Autodesk Inventor part; units mm, degrees
ref_plane "YZ Plane" through (0, 0, 0) normal (1, 0, 0) x (0, 1, 0)
ref_plane "XZ Plane" through (0, 0, 0) normal (0, 1, 0) x (-1, 0, 0)
ref_plane "XY Plane" through (0, 0, 0) normal (0, 0, 1) x (1, 0, 0)
sketch "Sketch1" plane through (0, 0, 0) normal (0, 1, 0) x (-1, 0, 0)
  line L0 (-30, -43) -> (30, -43)
  line L1 (30, -43) -> (30, 43)
  line L2 (30, 43) -> (-30, 43)
  line L3 (-30, 43) -> (-30, -43)
  line L4 (-30, -43) -> (30, 43) construction
  line L5 (30, -43) -> (-30, 43) construction
  line L6 (0, 43) -> (0, 45)
  line L7 (30, 0) -> (32, 0)
  line L8 (-30, -45) -> (30, -45)
  line L9 (32, -43) -> (32, 43)
  line L10 (30, 45) -> (-30, 45)
  line L11 (-32, 43) -> (-32, -43)
  line L12 (-32, -45) -> (32, 45) construction
  line L13 (32, -45) -> (-32, 45) construction
  arc A0 (-32, -43) -> (-30, -45) centre (-30, -43) ccw
  arc A1 (30, -45) -> (32, -43) centre (30, -43) ccw
  arc A2 (32, 43) -> (30, 45) centre (30, 43) ccw
  arc A3 (-30, 45) -> (-32, 43) centre (-30, 43) ccw
  point P0 (0, 0)
  dimension "d0" = 60
  dimension "d1" = 86
  dimension "d3" = 2
  dimension "d4" = 2
  dimension "d26" = 2
extrude "Extrusion1" add sketch "Sketch1" along normal blind 2
sketch "Sketch2" plane through (0, 2, 0) normal (0, 1, 0) x (1, 0, 0)
  line L0 (-30, -43) -> (30, -43)
  line L1 (30, -43) -> (30, 43)
  line L2 (30, 43) -> (-30, 43)
  line L3 (-30, 43) -> (-30, -43)
  line L4 (-30, -43) -> (30, 43) construction
  line L5 (30, -43) -> (-30, 43) construction
  line L6 (0, 43) -> (0, 45)
  line L7 (30, 0) -> (32, 0)
  line L8 (-30, -45) -> (30, -45)
  line L9 (32, -43) -> (32, 43)
  line L10 (30, 45) -> (-30, 45)
  line L11 (-32, 43) -> (-32, -43)
  line L12 (-32, -45) -> (32, 45) construction
  line L13 (32, -45) -> (-32, 45) construction
  arc A0 (32, 43) -> (30, 45) centre (30, 43) ccw
  arc A1 (-30, 45) -> (-32, 43) centre (-30, 43) ccw
  arc A2 (-32, -43) -> (-30, -45) centre (-30, -43) ccw
  arc A3 (30, -45) -> (32, -43) centre (30, -43) ccw
  point P0 (0, 0)
  point P1 (0, 0)
  dimension "d7" = 60
  dimension "d8" = 86
  dimension "d9" = 2
  dimension "d10" = 2
  dimension "d27" = 2
extrude "Extrusion2" add sketch "Sketch2" along normal blind 55 contours L0 L1 L7 L9 A3 L8 A2 L11 A1 L10 L6 L2 L3 | L1 L2 L6 L10 A0 L9 L7
sketch "Sketch3" plane through (32, 0, 45) normal (1, 0, 0) x (0, 0, -1)
  line L0 (2, 57) -> (88, 57)
  line L1 (2, 0) -> (88, 0)
  line L2 (107.729, 73.7861) -> (177.229, 73.7861)
  line L3 (106.879, 66.2861) -> (106.879, 57.2861)
  line L4 (106.879, 66.2861) -> (106.879, 72.9361)
  line L5 (106.879, 50.6361) -> (106.879, 57.2861)
  line L6 (177.229, 49.7861) -> (107.729, 49.7861)
  line L7 (178.079, 72.9361) -> (178.079, 50.6361)
  line L8 (142.479, 73.7861) -> (142.479, 49.7861)
  line L9 (178.079, 49.7861) -> (106.879, 49.7861)
  line L10 (106.879, 49.7861) -> (106.879, 73.7861)
  line L11 (106.879, 73.7861) -> (178.079, 73.7861)
  line L12 (178.079, 73.7861) -> (178.079, 49.7861)
  line L13 (178.079, 49.7861) -> (106.879, 73.7861) construction
  line L14 (106.879, 49.7861) -> (178.079, 73.7861) construction
  line L15 (177.069, 73.2861) -> (107.389, 73.2861)
  line L16 (82.6, 47) -> (52.1, 47)
  line L17 (7.6, 11) -> (82.6, 11)
  line L18 (7.6, 11) -> (82.6, 11)
  circle A0 centre (7.6, 44.5) radius 1.25
  line L19 (5.1, 44.5) -> (5.1, 13.5)
  line L20 (7.6, 11) -> (82.6, 11)
  line L21 (5.1, 11) -> (7.6, 11)
  circle A1 centre (7.6, 13.5) radius 1.25
  line L22 (5.1, 13.5) -> (5.1, 11)
  line L23 (82.6, 11) -> (85.1, 11)
  circle A2 centre (82.6, 13.5) radius 1.25
  circle A3 centre (82.6, 44.5) radius 1.25
  line L24 (85.1, 47) -> (82.6, 47)
  circle A4 centre (7.6, 44.5) radius 1.25
  line L25 (85.1, 47) -> (85.1, 11)
  line L26 (52.1, 47) -> (5.1, 47)
  line L27 (5.1, 47) -> (5.1, 44.5)
  line L28 (80.85, 17.25) -> (9.15, 17.25)
  line L29 (9.15, 17.25) -> (9.15, 41.75)
  line L30 (9.15, 41.75) -> (80.85, 41.75)
  line L31 (80.85, 41.75) -> (80.85, 17.25)
  line L32 (80.85, 17.25) -> (9.15, 41.75) construction
  line L33 (9.15, 17.25) -> (80.85, 41.75) construction
  point P0 (45, 0)
  point P1 (0, 57)
  point P2 (90, 57)
  point P3 (0, 0)
  point P4 (90, 0)
  point P5 (142.479, 61.7861)
  point P6 (45, 29.5)
  dimension "d21" = 71.7
  dimension "d22" = 24.5
  dimension "d100" = 2.5
extrude "Extrusion3" cut sketch "Sketch3" against normal blind 10 contours A0 | A1 | A2 | A3 | L28 L29 L30 L31
sketch "Sketch4" plane through (32, 0, -45) normal (0, 0, -1) x (-1, 0, 0)
  line L0 (32, 0) -> (32, 12.5)
  line L1 (32, 12.5) -> (39.5, 12.5)
  line L2 (40.5, 13.5) -> (40.5, 17.5)
  line L3 (39.5, 18.5) -> (32, 18.5)
  line L4 (32, 18.5) -> (32, 12.5)
  line L5 (32, 12.5) -> (24.5, 12.5)
  line L6 (23.5, 13.5) -> (23.5, 17.5)
  line L7 (24.5, 18.5) -> (32, 18.5)
  arc A0 (24.5, 18.5) -> (23.5, 17.5) centre (24.5, 17.5) ccw
  arc A1 (23.5, 13.5) -> (24.5, 12.5) centre (24.5, 13.5) ccw
  arc A2 (39.5, 12.5) -> (40.5, 13.5) centre (39.5, 13.5) ccw
  arc A3 (40.5, 17.5) -> (39.5, 18.5) centre (39.5, 17.5) ccw
  point P0 (40.5, 18.5)
  point P1 (40.5, 12.5)
  point P2 (23.5, 18.5)
  point P3 (23.5, 12.5)
  dimension "d23" = 12.5
  dimension "d24" = 8.5
  dimension "d25" = 6
  dimension "d28" = 1
extrude "Extrusion4" cut sketch "Sketch4" against normal blind 10
sketch "Sketch5" plane through (-32, 0, -43) normal (-1, 0, 0) x (0, 0, 1)
  line L0 (0, 2) -> (86, 2)
  line L1 (86, 2) -> (66, 2)
  line L2 (66, 17) -> (72.05, 17)
  line L3 (66, 17) -> (59.95, 17)
  line L4 (58.95, 18) -> (58.95, 28)
  line L5 (59.95, 29) -> (72.05, 29)
  line L6 (73.05, 28) -> (73.05, 18)
  arc A0 (59.95, 29) -> (58.95, 28) centre (59.95, 28) ccw
  arc A1 (73.05, 28) -> (72.05, 29) centre (72.05, 28) ccw
  arc A2 (58.95, 18) -> (59.95, 17) centre (59.95, 18) ccw
  arc A3 (72.05, 17) -> (73.05, 18) centre (72.05, 18) ccw
  line L7 (66, 29) -> (66, 17)
  line L8 (66, 23) -> (58.95, 23)
  line L9 (78.85, 17.25) -> (7.15, 17.25)
  line L10 (66, 17) -> (67, 17) construction
  line L11 (15, 17) -> (16, 17)
  line L12 (17, 17) -> (12, 17)
  line L13 (11.5, 17.5) -> (11.5, 22.5)
  line L14 (12, 23) -> (17, 23)
  line L15 (17.5, 22.5) -> (17.5, 17.5)
  arc A4 (11.5, 17.5) -> (12, 17) centre (12, 17.5) ccw
  arc A5 (17, 17) -> (17.5, 17.5) centre (17, 17.5) ccw
  arc A6 (12, 23) -> (11.5, 22.5) centre (12, 22.5) ccw
  arc A7 (17.5, 22.5) -> (17, 23) centre (17, 22.5) ccw
  point P0 (43, 0)
  point P1 (73.05, 17)
  point P2 (58.95, 17)
  point P3 (58.95, 29)
  point P4 (14.5, 20)
  point P5 (17.5, 20)
  point P6 (11.5, 23)
  point P7 (11.5, 17)
  point P8 (17.5, 23)
  point P9 (11.567, 17.25)
  point P10 (17.433, 17.25)
  dimension "d31" = 20
  dimension "d32" = 15
  dimension "d33" = 7.05
  dimension "d34" = 12
  dimension "d35" = 1
  dimension "d83" = 50
  dimension "d89" = 6
  dimension "d90" = 6
  dimension "d91" = 0.5
extrude "Extrusion5" cut sketch "Sketch5" against normal blind 10 contours L7 L9 A3 L2 | L9 A4 L13 A6 L14 A7 L15 A5 | L3 A2 L9 L7 | L9 A2 L4 L8 L7 | L7 L5 A1 L6 A3 L9 | L8 L4 A0 L5 L7
sketch "Sketch6" plane through (-30, 2, 43) normal (1, 0, 0) x (0, 0, -1)
  line L0 (0, 55) -> (86, 55)
  line L1 (43, 55) -> (43, 48)
  line L2 (43, 48) -> (39.5, 48)
  line L3 (39.5, 48) -> (39.5, 55)
  line L4 (43, 48) -> (46.5, 48)
  line L5 (46.5, 48) -> (46.5, 55)
  point P0 (43, -2)
  dimension "d38" = 7
  dimension "d39" = 3.5
extrude "Extrusion6" add sketch "Sketch6" along normal blind 7
sketch "Sketch8" plane through (-30, 50, 3.5) normal (0, 0, 1) x (1, 0, 0)
  line L0 (7, 7) -> (7, 0)
  line L1 (0, 0) -> (7, 0)
  line L2 (0, 0) -> (0, 7)
  line L3 (0, 7) -> (7, 7)
  line L4 (7, 7) -> (0, 0)
  point P0 (30, -50)
extrude "Extrusion7" cut sketch "Sketch8" against normal blind 7 contours L0 L1 L4
sketch "Sketch9" plane through (0, 57, 0) normal (0, 1, 0) x (1, 0, 0)
  line L0 (-30, 3.5) -> (-23, 3.5)
  line L1 (-30, -3.5) -> (-23, -3.5)
  line L2 (-23, 3.5) -> (-23, -3.5)
  line L3 (-30, 3.5) -> (-30, -3.5)
  line L4 (-30, 43) -> (-30, -43)
  line L5 (-23, 0) -> (-28, 0)
  circle A0 centre (-28, 0) radius 1.5
  point P0 (0, 0)
  dimension "d47" = 5
  dimension "d48" = 3
extrude "Extrusion8" cut sketch "Sketch9" against normal blind 3 contours A0
sketch "Sketch11" plane through (-30, 2, -43) normal (0, 0, 1) x (1, 0, 0)
  line L0 (0, 55) -> (60, 55)
  line L1 (30, 55) -> (30, 48)
  line L2 (30, 48) -> (33.5, 48)
  line L3 (33.5, 48) -> (33.5, 55)
  line L4 (30, 48) -> (26.5, 48)
  line L5 (26.5, 48) -> (26.5, 55)
  point P0 (30, -2)
  dimension "d49" = 7
  dimension "d50" = 3.5
  dimension "d51" = 3.5
extrude "Extrusion9" add sketch "Sketch11" along normal blind 7
sketch "Sketch12" plane through (-3.5, 50, -43) normal (-1, 0, 0) x (0, 0, 1)
  line L0 (7, 7) -> (7, 0)
  line L1 (0, 0) -> (7, 0)
  line L2 (7, 7) -> (0, 0)
  point P0 (43, -50)
extrude "Extrusion10" cut sketch "Sketch12" against normal blind 7
sketch "Sketch13" plane through (0, 57, 0) normal (0, 1, 0) x (1, 0, 0)
  line L0 (3.5, 36) -> (-3.5, 36)
  line L1 (0, 36) -> (0, 41)
  circle A0 centre (0, 41) radius 1.5
  point P0 (0, 0)
  dimension "d56" = 5
  dimension "d57" = 3
extrude "Extrusion11" cut sketch "Sketch13" against normal blind 3
sketch "Sketch14" plane through (30, 2, -43) normal (-1, 0, 0) x (0, 0, 1)
  line L0 (0, 55) -> (86, 55)
  line L1 (43, 55) -> (43, 48)
  line L2 (43, 48) -> (46.5, 48)
  line L3 (46.5, 48) -> (46.5, 55)
  line L4 (43, 48) -> (39.5, 48)
  line L5 (39.5, 48) -> (39.5, 55)
  point P0 (43, -2)
  dimension "d60" = 7
  dimension "d61" = 3.5
extrude "Extrusion12" add sketch "Sketch14" along normal blind 7
sketch "Sketch17" plane through (30, 50, -3.5) normal (0, 0, -1) x (-1, 0, 0)
  line L0 (7, 7) -> (7, 0)
  line L1 (0, 0) -> (7, 0)
  line L2 (0, 0) -> (7, 7)
  point P0 (30, -50)
extrude "Extrusion13" cut sketch "Sketch17" against normal blind 7
sketch "Sketch18" plane through (0, 57, 0) normal (0, 1, 0) x (1, 0, 0)
  line L0 (23, -3.5) -> (23, 3.5)
  line L1 (23, 0) -> (28, 0)
  circle A0 centre (28, 0) radius 1.5
  point P0 (0, 0)
  dimension "d66" = 5
  dimension "d67" = 3
extrude "Extrusion14" cut sketch "Sketch18" against normal blind 3
sketch "Sketch19" plane through (30, 2, 43) normal (0, 0, -1) x (-1, 0, 0)
  line L0 (0, 55) -> (60, 55)
  line L1 (30, 55) -> (30, 48)
  line L2 (30, 48) -> (33.5, 48)
  line L3 (33.5, 48) -> (33.5, 55)
  line L4 (30, 48) -> (26.5, 48)
  line L5 (26.5, 48) -> (26.5, 55)
  point P0 (30, -2)
  dimension "d70" = 7
  dimension "d71" = 3.5
extrude "Extrusion15" add sketch "Sketch19" along normal blind 7
sketch "Sketch20" plane through (3.5, 50, 43) normal (1, 0, 0) x (0, 0, -1)
  line L0 (7, 7) -> (7, 0)
  line L1 (0, 0) -> (7, 0)
  line L2 (0, 0) -> (7, 7)
  point P0 (43, -50)
extrude "Extrusion16" cut sketch "Sketch20" against normal blind 7
sketch "Sketch21" plane through (0, 57, 0) normal (0, 1, 0) x (1, 0, 0)
  line L0 (-3.5, -36) -> (3.5, -36)
  line L1 (-3.5, -43) -> (-3.5, -36)
  line L2 (3.5, -43) -> (3.5, -36)
  line L3 (0, -36) -> (0, -41)
  circle A0 centre (0, -41) radius 1.5
  point P0 (0, 0)
  dimension "d76" = 5
  dimension "d77" = 3
extrude "Extrusion17" cut sketch "Sketch21" against normal blind 3
sketch "Sketch23" plane through (-30, 0, 45) normal (0, 0, 1) x (1, 0, 0)
  line L0 (0, 2) -> (60, 2)
  line L1 (0, 57) -> (60, 57)
  line L2 (30, 2) -> (30, 12)
  circle A0 centre (30, 32) radius 1.65
  line L3 (32.5, 9) -> (27.5, 9)
  line L4 (27, 9.5) -> (27, 14.5)
  line L5 (27.5, 15) -> (32.5, 15)
  line L6 (33, 14.5) -> (33, 9.5)
  line L7 (33, 9) -> (27, 15) construction
  line L8 (27, 9) -> (33, 15) construction
  arc A1 (33, 14.5) -> (32.5, 15) centre (32.5, 14.5) ccw
  arc A2 (27.5, 15) -> (27, 14.5) centre (27.5, 14.5) ccw
  arc A3 (27, 9.5) -> (27.5, 9) centre (27.5, 9.5) ccw
  arc A4 (32.5, 9) -> (33, 9.5) centre (32.5, 9.5) ccw
  point P0 (30, 0)
  dimension "d92" = 10
  dimension "d94" = 3.3
  dimension "d95" = 6
  dimension "d96" = 6
  dimension "d97" = 0.5
extrude "Extrusion18" cut sketch "Sketch23" against normal blind 10
properties part number "Case Bottom"
Model file for the job. Use its own axes, mm. A direction names the side the tool comes from. Round coordinates to 2 decimals unless told otherwise and drop trailing zeros. Order: outer loops, then holes, each group sorted by start corner. A loop starts at its lowest first (then second) coordinate and runs counter-clockwise, first axis right, second up.
(1) Pin check, flat tips, straight feed: pin 1 (1.8 mm diameter, centred on x = 0, z = 41, fed in from +Y); pin 2 (8 mm diameter, centred on x = -18, z = -9.5, fed in from +Y); pin 3 (1 mm diameter, centred on x = -31.5, y = 20, fed in from -Z); pin 4 (6 mm diameter, centred on y = 24, z = 23, fed in from -X). Stop position of each tip, or through.
(2) Band-saw the part on A-A (x = 5.5). List the corners of the cut face in (y, z).
(3) 3-axis set-ups, long thin cutter, end or side, ignore diameter. For faces 4 (the face through (31, 29, 35.85)), 5 (the face through (-31, 17, 23)), 6 (the face through (-3.5, 55, 41)), 7 (the face through (3, 12, 44)): which of +Z, -Z, +X, -X, +Y, -Y reach the whole face in a straight line?
(4) Pull direction Y, two halves, no side cores. Call faces 1 (the face through (0, 54, 41)), 2 (the face through (-0.325, 55.521, 42.464)), 3 (the face through (31, 17.25, -1)): released by +Y, released by -Y, zero draft, split by the parting line, or undercut.
(5) Band-saw the part on D-D (z = 0). List the corners of the cut face in (x, y), then the cut area to 3 significant figures.
(6) Band-saw the part on B-B (y = 44.5). List the corners of the cut face in (x, z).
(7) Drill centre lines: line 1 (Y direction, x = 31.3, z = 37.4); line 2 (Z direction, x = -8.5, y = 50); line 3 (X direction, y = 11, z = -3.5). Where is each one in solid material? Low to high.
(8) Band-saw the part on C-C (z = -27.5). List the corners of the cut face in (x, y).
Verdict:
1. pin 1: stops at y = 54
1. pin 2: stops at y = 2
1. pin 3: stops at z = -44.73
1. pin 4: passes through
2. outline: (0, -45) - (12.5, -45) - (12.5, -43) - (2, -43) - (2, 43) - (57, 43) - (57, 45) - (0, 45) - close; (18.5, -45) - (57, -45) - (57, -43) - (18.5, -43) - close
3. face 4: +X
3. face 5: -X
3. face 6: +Y
3. face 7: +Z
4. face 1: released by +Y
4. face 2: zero draft
4. face 3: undercut
5. outline: (-32, 0) - (32, 0) - (32, 17.25) - (30, 17.25) - (30, 2) - (-30, 2) - (-30, 50) - (-23, 57) - (-26.5, 57) - (-26.5, 54) - (-29.5, 54) - (-29.5, 57) - (-32, 57) - close; (23, 57) - (30, 50) - (30, 41.75) - (32, 41.75) - (32, 57) - (29.5, 57) - (29.5, 54) - (26.5, 54) - (26.5, 57) - close
5. area: 330 mm2
6. outline: (-32, -43) arc R2 ccw to (-30, -45) - (30, -45) arc R2 ccw to (32, -43) - (32, -38.85) - (30, -38.85) - (30, -43) - (-30, -43) - (-30, 43) - (30, 43) - (30, 38.65) - (32, 38.65) - (32, 43) arc R2 ccw to (30, 45) - (-30, 45) arc R2 ccw to (-32, 43) - close; (30, -36.35) - (32, -36.35) - (32, 36.15) - (30, 36.15) - close
7. line 1: y = 0 to 12.25, 14.75 to 43.25, 45.75 to 57
7. line 2: z = -45 to -43, 43 to 45
7. line 3: x = -32 to -30, 30 to 32
8. outline: (-32, 0) - (32, 0) - (32, 17.25) - (30, 17.25) - (30, 2) - (-30, 2) - (-30, 17.25) - (-32, 17.25) - close; (-32, 23) - (-30, 23) - (-30, 57) - (-32, 57) - close; (30, 41.75) - (32, 41.75) - (32, 57) - (30, 57) - close
